Geometry check sheet. Reference: the model listing, model coordinates, mm. A direction names the side the tool comes from. Round coordinates to 2 decimals unless told otherwise and drop trailing zeros. Write each loop counter-clockwise with the first axis right and the second up, starting at its lowest first coordinate (ties: lowest second). Pieces come first, ordered by that corner, then holes.
Item 1: Access from +Z, -Z, +X, -X, +Y, -Y to the whole of each face (thin tool, end or side, straight path). Record for faces 1 (the face through (-26, 0, -51)), 2 (the face through (-14, -3, -49.891)), 3 (the face through (3, -2, -56.217)).
Item 2: Cross-section at A-A (z = 0). Enter the section's corners in (x, y), then the cut area to 3 significant figures.
Item 3: Cross-section at B-B (x = 43). Enter the section's corners in (y, z), then the cut area to 3 significant figures.
Item 4: Scan lines: probe 1 along Z at (x, y) = (-8, -1); probe 2 along Y at (x, z) = (33, -3.5); probe 3 along X at (y, z) = (3.5, 10). Record each from-to range of solid material in increasing order.
Item 5: Depth check by flat-ended pin: P1, Ø2, axis at x = -43, z = -15, coming from the +Y side; P2, Ø1.6, axis at x = 55.5, z = -4, coming from the -Y side; P3, Ø6, axis at x = -33.5, z = 29.5, coming from the +Y side. Enter the tip coordinate at first touch or a pass-through.
Item 6: Cross-section at C-C (y = 4). Enter the section's corners in (x, z), then the cut area to 3 significant figures.
Item 7: Draft check along Z on faces 4 (the face through (57.04, 25, -9)), 5 (the face through (3, -2, 39.121)), 6 (the face through (-14, -8.382, -8)). Enter one of: pulls with the +Z half, pulls with the -Z half, needs draft (parallel to the pull), parting line crosses it, or undercut.
from build123d import *

# Parameters (mm, degrees)
F0_W     = 144.580562
F0_H     = 95.337302
F0_W_2   = 134.136807
F0_H_2   = 82.360171
F1_DEPTH = 8.382
F2_W     = 64.001322
F2_H     = 95.337302
F2_W_2   = 49.989581
F2_H_2   = 82.352217
F3_DEPTH = 4.572
F4_SIZE  = 2.54
F5_W     = 50.907161
F5_H     = 84.29788
F6_DEPTH = 2.032
F7_SIZE  = 2.54
F8_W     = 136.117357
F8_H     = 84.297877
F9_DEPTH = 2.286


with BuildPart() as f1:
    # F0 (on Front) → F1 (new body)
    with BuildSketch(Plane.XZ):
        with Locations((-13.217857, -8.547984)):
            Rectangle(F0_W, F0_H)
        with Locations((-13.217868, -8.711174)):
            Rectangle(F0_W_2, F0_H_2, mode=Mode.SUBTRACT)
    extrude(amount=F1_DEPTH)

    # F2 (on face) → F3 (join)
    with BuildSketch(Plane.YZ.offset(59.072424)):
        with Locations((23.618661, -8.547984)):
            Rectangle(F2_W, F2_H)
        with Locations((24.994791, -9.356501)):
            Rectangle(F2_W_2, F2_H_2, mode=Mode.SUBTRACT)
    extrude(amount=-F3_DEPTH)

    # F4
    f4_edges = [f1.edges().sort_by_distance(p)[0] for p in [
        (59.072424, 0, -9.356501),
        (59.072424, 24.994791, 31.819608),
        (59.072424, 49.989581, -9.356501),
        (59.072424, 24.994791, -50.532609),
    ]]
    chamfer(f4_edges, length=F4_SIZE)

    # F5 (on face) → F6 (join)
    with BuildSketch(Plane.YZ.offset(59.072424)):
        with Locations((25.45358, -9.214379)):
            Rectangle(F5_W, F5_H)
    extrude(amount=-F6_DEPTH)

    # F7
    f7_edges = [f1.edges().sort_by_distance(p)[0] for p in [
        (-13.217868, -8.382, 32.468911),
        (-80.286272, -8.382, -8.711174),
        (-13.217868, -8.382, -49.89126),
        (53.850535, -8.382, -8.711174),
    ]]
    chamfer(f7_edges, length=F7_SIZE)

    # F8 (on face) → F9 (join)
    with BuildSketch(Plane.XZ.offset(8.382)):
        with Locations((-13.412287, -8.484526)):
            Rectangle(F8_W, F8_H)
    extrude(amount=-F9_DEPTH)


solid = f1.part
Resolved:
1. face 1: +Z, -Z, -X, +Y
1. face 2: +Y
1. face 3: -Z, +X, -X, +Y, -Y
2. outline: (-85.51, -8.38) - (-82.83, -8.38) - (-81.47, -7.03) - (-81.47, -8.38) - (54.65, -8.38) - (54.65, -6.64) - (56.39, -8.38) - (59.07, -8.38) - (59.07, -2.54) - (56.53, 0) - (53.85, 0) - (53.85, -5.84) - (54.1, -6.1) - (-80.54, -6.1) - (-80.29, -5.84) - (-80.29, 0) - (-85.51, 0) - close; (54.5, 49.99) - (56.53, 49.99) - (57.04, 50.5) - (57.04, 0) - (59.07, 0) - (59.07, 50.91) - (57.45, 50.91) - (59.07, 52.53) - (59.07, 55.62) - (54.5, 55.62) - close
2. area: 514 mm2
3. outline: (-8.38, -56.22) - (0, -56.22) - (0, -49.89) - (-5.84, -49.89) - (-6.1, -50.15) - (-6.1, 32.72) - (-5.84, 32.47) - (0, 32.47) - (0, 39.12) - (-8.38, 39.12) - (-8.38, 35.01) - (-7.04, 33.66) - (-8.38, 33.66) - (-8.38, -50.63) - (-6.58, -50.63) - (-8.38, -52.43) - close
3. area: 294 mm2
4. probe 1: z = -56.22 to -49.89, 32.47 to 39.12
4. probe 2: y = -8.38 to -6.1
4. probe 3: x = 57.04 to 59.07
5. P1: stops at y = -6.1
5. P2: stops at y = -8.29
5. P3: stops at y = 0
6. outline: (54.5, -56.22) - (59.07, -56.22) - (59.07, -53.07) - (57.36, -51.36) - (59.07, -51.36) - (59.07, 32.93) - (57.65, 32.93) - (59.07, 34.36) - (59.07, 39.12) - (54.5, 39.12) - (54.5, 31.82) - (56.53, 31.82) - (57.04, 32.33) - (57.04, -51.04) - (56.53, -50.53) - (54.5, -50.53) - close
6. area: 224 mm2
7. face 4: undercut
7. face 5: pulls with the +Z half
7. face 6: needs draft
